```python
from build123d import *

# Parameters (mm, degrees)
SKETCH1_R            = 1.25
EXTRUDE1_DEPTH       = 6
CUT_SWEEP1_PITCH     = 0.45
SKETCH6_R            = 2.25
EXTRUDE2_DEPTH       = 2.5
CUT_EXTRUDE1_DEPTH   = 1.5
CHAMFER1_SIZE        = 0.225
SKETCH10_R           = 1.25
PARTIAL_THREAD_DEPTH = 6
CHAMFER2_SIZE        = 0.05


with BuildPart() as part:
    # Sketch1 → Extrude1 (new body)
    with BuildSketch(Plane.XY):
        Circle(SKETCH1_R)
    extrude(amount=-EXTRUDE1_DEPTH)

    # Cut-Sweep1: arcs per turn and ends read off the stored shape
    # Cut-Sweep1: the profile of Sketch3 profile screwed along a right-hand helix through 16 turns, 6 arcs to a turn; built about Z, then put on its axis
    cut_sweep1_z = Axis((0, 0, 0), (0, 0, 1))
    cut_sweep1_corners = [(1.2503, 0, -0.843923205), (0.957716426, 0, -0.675), (0.957716426, 0, -0.61875), (1.2503, 0, -0.449826795)]
    with BuildLine(mode=Mode.PRIVATE) as cut_sweep1_profile:
        Line(cut_sweep1_corners[0], cut_sweep1_corners[1])
        Line(cut_sweep1_corners[1], cut_sweep1_corners[2])
        Line(cut_sweep1_corners[2], cut_sweep1_corners[3])
        Line(cut_sweep1_corners[3], cut_sweep1_corners[0])
    cut_sweep1_cap = Face(cut_sweep1_profile.wire())
    cut_sweep1_turn_angles = [0, 30, 60, 90, 120, 150, 180, 210, 240, 270, 300, 330, 360]
    cut_sweep1_turn_weights = [1, 0.8660254037844387, 1, 0.8660254037844387, 1, 0.8660254037844387, 1, 0.8660254037844387, 1, 0.8660254037844387, 1, 0.8660254037844387, 1]
    cut_sweep1_turn_rails = [Edge.make_bspline([Vector(p[0], p[1], 0).rotate(cut_sweep1_z, cut_sweep1_turn_angles[k]) / cut_sweep1_turn_weights[k] + Vector(0, 0, p[2] + CUT_SWEEP1_PITCH * cut_sweep1_turn_angles[k] / 360) for k in range(13)], [0, 0, 0, 1, 1, 2, 2, 3, 3, 4, 4, 5, 5, 6, 6, 6], 2, cut_sweep1_turn_weights) for p in cut_sweep1_corners]
    cut_sweep1_turn_sides = [Face.make_surface_from_curves(cut_sweep1_turn_rails[p[0]], cut_sweep1_turn_rails[p[1]]) for p in [(0, 1), (1, 2), (2, 3), (3, 0)]]
    cut_sweep1 = Plane(origin=(0, 0, 0), x_dir=(0, 1, 0), z_dir=(0, 0, -1)) * Solid(Shell([*[p.moved(Location((0, 0, CUT_SWEEP1_PITCH * i))) for i in range(16) for p in cut_sweep1_turn_sides], cut_sweep1_cap, cut_sweep1_cap.rotate(cut_sweep1_z, 5760).moved(Location((0, 0, CUT_SWEEP1_PITCH * 5760 / 360)))]))
    add(cut_sweep1, mode=Mode.SUBTRACT)

    # Sketch4 → Cut-Revolve1 (revolve, cut)
    with BuildSketch(Plane(origin=(0, 0, 0), x_dir=(0, 0, -1), z_dir=(1, 0, 0)), mode=Mode.PRIVATE) as cut_revolve1_sk:
        Polygon((0.382511876, 1.25), (0, 0.703716426), (0, 1.25), align=None)
    revolve(cut_revolve1_sk.sketch.rotate(Axis((0, 0, 0), (0, 0, -1)), 270), axis=Axis((0, 0, 0), (0, 0, -1)), mode=Mode.SUBTRACT)

    # Sketch6 → Extrude2 (add)
    with BuildSketch(Plane(origin=(0, 0, -6), x_dir=(-1, 0, 0), z_dir=(0, 0, -1))):
        Circle(SKETCH6_R)
    extrude(amount=EXTRUDE2_DEPTH)

    # Sketch7 → Cut-Extrude1 (cut)
    with BuildSketch(Plane(origin=(0, 0, -8.5), x_dir=(-1, 0, 0), z_dir=(0, 0, -1))):
        Polygon((0, 1.154700538), (-1, 0.577350269), (-1, -0.577350269), (0, -1.154700538), (1, -0.577350269), (1, 0.577350269), align=None)
    extrude(amount=-CUT_EXTRUDE1_DEPTH, mode=Mode.SUBTRACT)

    # Cut-Extrude2 cone 1 section (through the dimple's axis) → Cut-Extrude2 (revolve, cut)
    with BuildSketch(Plane(origin=(0, 0, -8.5), x_dir=(0, 1, 0), z_dir=(1, 0, 0))):
        Polygon((0, 0), (1.154700538, 0), (0, 1.154700538), align=None)
    revolve(axis=Axis((0, 0, -8.5), (0, 0, 1)), mode=Mode.SUBTRACT)

    # Chamfer1
    chamfer1_edges = [part.edges().sort_by_distance(p)[0] for p in [
        (2.25, 0, -6),
        (2.25, 0, -8.5),
    ]]
    chamfer(chamfer1_edges, length=CHAMFER1_SIZE)


with BuildPart() as body_2:
    # Sketch10 → partial thread (new body)
    with BuildSketch(Plane.XY.offset(-6)):
        Circle(SKETCH10_R)
    extrude(amount=PARTIAL_THREAD_DEPTH)

    # Chamfer2
    chamfer2_edges = [body_2.edges().sort_by_distance(p)[0] for p in [
        (-1.25, 0, 0),
    ]]
    chamfer(chamfer2_edges, length=CHAMFER2_SIZE)


with BuildPart() as part_1:
    add(part.part)

    # Combine1: union body 2
    add(body_2.part)


solid = part_1.part
```
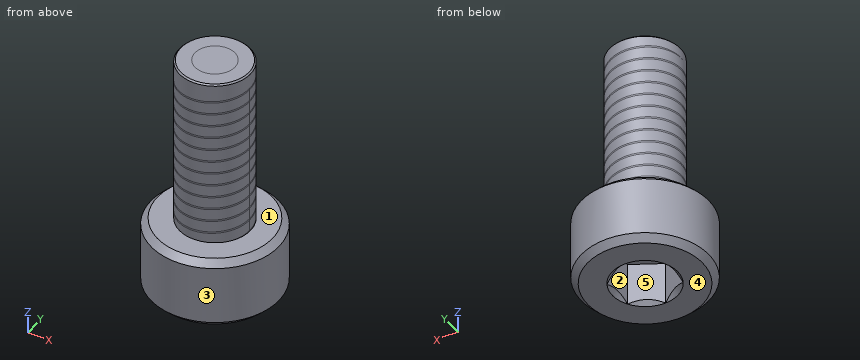
Part model, mm, in its own coordinate system. Face numbers are marked on the shaded views. A direction names the side the tool comes from. Round coordinates to 2 decimals unless told otherwise and drop trailing zeros. Loops run counter-clockwise (first coordinate to the right, second up) from the corner with the lowest first, then second, coordinate; pieces in that order, holes last.
1. Two-plate mould, pull along X, no slides. Class the marked faces 1, 2 and 3: pulls with the +X half, pulls with the -X half, needs draft (parallel to the pull), parting line crosses it, or undercut.
Solutions:
face 1: needs draft
face 2: undercut
face 3: parting line crosses it
2. 3-axis set-ups, long thin cutter, end or side, ignore diameter. For the marked faces 4 and 5: which of +Z, -Z, +X, -X, +Y, -Y reach the whole face in a straight line?
Solutions:
face 4: -Z, +X, -X, +Y, -Y
face 5: -Z
3. Slice it at A-A (z = -6.5). Give the cut face in (x, y).
Solutions:
outline: circle Ø4.5 at (0, 0)
4. Slice it at B-B (z = -1.25). Give the cut face in (x, y).
Solutions:
outline: circle Ø2.5 at (0, 0)
5. Flat gauge pins, fed straight in: pin 1 (1 mm diameter, centred on x = -1.5, z = -6, fed in from +Y); pin 2 (1 mm diameter, centred on x = 1.5, y = -1.5, fed in from +Z); pin 3 (1 mm diameter, centred on x = 0, y = -0.5, fed in from -Z). Where does each tip first touch, or does it go through?
Solutions:
pin 1: stops at y = 1.99
pin 2: stops at z = -6
pin 3: stops at z = -7
6. Drill centre lines: line 1 along Z through (x, y) = (-0.8, -1.2); line 2 along Z through (x, y) = (-0.3, -0.2); line 3 along Y through (x, z) = (-0.9, -7.5). Where is each one in solid material? Low to high.
Solutions:
line 1: z = -8.5 to -6
line 2: z = -7 to 0
line 3: y = -2.06 to -0.64, 0.64 to 2.06
